```python
from build123d import *

# Parameters (mm, degrees)
SKETCH1_W            = 213.868
SKETCH1_H            = 49.53
BOSS_EXTRUDE1_DEPTH  = 63.5
SKETCH2_W            = 203.708
SKETCH2_H            = 39.37
CUT_EXTRUDE1_DEPTH   = 11.43
SKETCH3_W            = 191.008
SKETCH3_H            = 29.21
CUT_EXTRUDE2_DEPTH   = 45.72
SKETCH5_W            = 29.21
SKETCH5_H            = 45.72
BOSS_EXTRUDE2_DEPTH  = 31.75
SKETCH7_W            = 29.21
SKETCH7_H            = 45.802108617
BOSS_EXTRUDE3_DEPTH  = 31.75
BOSS_EXTRUDE4_DEPTH  = 40.64
BOSS_EXTRUDE5_DEPTH  = 40.64
SKETCH20_W           = 12.7
SKETCH20_H           = 29.21
BOSS_EXTRUDE6_DEPTH  = 18.542
BOSS_EXTRUDE7_DEPTH  = 30.48
SKETCH22_W           = 106.68
SKETCH22_H           = 63.5
BOSS_EXTRUDE8_DEPTH  = 26.67
CUT_EXTRUDE11_DEPTH  = 96.52
CUT_EXTRUDE5_DEPTH   = 49.53
SKETCH28_W           = 12.7
SKETCH28_H           = 29.21
CUT_EXTRUDE6_DEPTH   = 28.702
BOSS_EXTRUDE9_DEPTH  = 29.21
SKETCH30_W           = 12.7
SKETCH30_H           = 29.21
CUT_EXTRUDE7_DEPTH   = 28.702
BOSS_EXTRUDE11_DEPTH = 29.21
BOSS_EXTRUDE12_DEPTH = 29.21
CUT_EXTRUDE8_DEPTH   = 49.53
BOSS_EXTRUDE13_DEPTH = 29.21
CUT_EXTRUDE9_DEPTH   = 50.8
CUT_EXTRUDE12_DEPTH  = 49.53
SKETCH48_W           = 12.7
SKETCH48_H           = 5.334
BOSS_EXTRUDE14_DEPTH = 31.242
BOSS_EXTRUDE17_DEPTH = 31.242
SKETCH52_W           = 12.7
SKETCH52_H           = 5.334
BOSS_EXTRUDE18_DEPTH = 31.242
BOSS_EXTRUDE19_DEPTH = 31.242
SKETCH54_W           = 12.7
SKETCH54_H           = 5.334
BOSS_EXTRUDE20_DEPTH = 31.242
BOSS_EXTRUDE21_DEPTH = 31.242
SKETCH56_W           = 12.7
SKETCH56_H           = 5.334
BOSS_EXTRUDE22_DEPTH = 31.242
BOSS_EXTRUDE23_DEPTH = 31.242


with BuildPart() as part:
    # Sketch1 → Boss-Extrude1 (new body)
    with BuildSketch(Plane(origin=(0, 0, 0), x_dir=(1, 0, 0), z_dir=(0, 1, 0))):
        with Locations((47.373649513, -17.485904033)):
            Rectangle(SKETCH1_W, SKETCH1_H)
    extrude(amount=BOSS_EXTRUDE1_DEPTH)

    # Sketch2 → Cut-Extrude1 (cut)
    with BuildSketch(Plane(origin=(0, 63.5, 0), x_dir=(1, 0, 0), z_dir=(0, 1, 0))):
        with Locations((47.373649513, -17.485904033)):
            Rectangle(SKETCH2_W, SKETCH2_H)
    extrude(amount=-CUT_EXTRUDE1_DEPTH, mode=Mode.SUBTRACT)

    # Sketch3 → Cut-Extrude2 (cut)
    with BuildSketch(Plane(origin=(0, 52.07, 0), x_dir=(1, 0, 0), z_dir=(0, 1, 0))):
        with Locations((47.373649513, -17.485904033)):
            Rectangle(SKETCH3_W, SKETCH3_H)
    extrude(amount=-CUT_EXTRUDE2_DEPTH, mode=Mode.SUBTRACT)

    # Sketch5 → Boss-Extrude2 (add)
    with BuildSketch(Plane.ZY.offset(-142.877649513)):
        with Locations((17.485904033, 29.21)):
            Rectangle(SKETCH5_W, SKETCH5_H)
    extrude(amount=BOSS_EXTRUDE2_DEPTH)

    # Sketch7 → Boss-Extrude3 (add)
    with BuildSketch(Plane(origin=(-48.130350487, 0, 0), x_dir=(0, 0, -1), z_dir=(1, 0, 0))):
        with Locations((-17.485904033, 29.168945691)):
            Rectangle(SKETCH7_W, SKETCH7_H)
    extrude(amount=BOSS_EXTRUDE3_DEPTH)

    # Sketch13 → Boss-Extrude4 (add)
    with BuildSketch(Plane.XY.offset(-2.199095967)):
        Polygon((-54.480350487, 62.738), (-48.130350487, 52.07), (-54.480350487, 52.07), align=None)
    extrude(amount=BOSS_EXTRUDE4_DEPTH)

    # Sketch19 → Boss-Extrude5 (add)
    with BuildSketch(Plane(origin=(0, 0, 37.170904033), x_dir=(-1, 0, 0), z_dir=(0, 0, -1))):
        Polygon((-149.227649513, 62.738), (-142.877649513, 52.07), (-149.227649513, 52.07), align=None)
    extrude(amount=BOSS_EXTRUDE5_DEPTH)

    # Sketch20 → Boss-Extrude6 (add)
    with BuildSketch(Plane(origin=(0, 6.35, 0), x_dir=(1, 0, 0), z_dir=(0, 1, 0))):
        with Locations((47.373649513, -17.485904033)):
            Rectangle(SKETCH20_W, SKETCH20_H)
    extrude(amount=BOSS_EXTRUDE6_DEPTH)

    # Sketch21 → Boss-Extrude7 (add)
    with BuildSketch(Plane.XY.offset(2.880904033)):
        Polygon((66.423649513, 37.592), (28.323649513, 37.592), (33.403649513, 24.892), (41.023649513, 24.892), (53.723649513, 24.892), (61.343649513, 24.892), align=None)
    extrude(amount=BOSS_EXTRUDE7_DEPTH)

    # Sketch22 → Boss-Extrude8 (add)
    with BuildSketch(Plane(origin=(0, 0, -7.279095967), x_dir=(-1, 0, 0), z_dir=(0, 0, -1))):
        with Locations((-46.357649513, 31.75)):
            Rectangle(SKETCH22_W, SKETCH22_H)
    extrude(amount=BOSS_EXTRUDE8_DEPTH)

    # Sketch39 → Cut-Extrude11 (cut)
    with BuildSketch(Plane(origin=(99.697649513, 0, 0), x_dir=(0, 0, -1), z_dir=(1, 0, 0))):
        with BuildLine():
            Line((12.359095967, 50.8), (12.359095967, 6.35))
            Line((12.359095967, 6.35), (27.599095967, 6.35))
            Line((27.599095967, 6.35), (27.599095967, 50.8))
            add(Edge.make_bspline(
                [(12.359095967, 50.8), (19.979095967, 66.04), (27.599095967, 50.8)],
                knots=[0, 0, 0, 1, 1, 1], degree=2))
        make_face()
    extrude(amount=-CUT_EXTRUDE11_DEPTH, mode=Mode.SUBTRACT)

    # Sketch26 → Cut-Extrude5 (cut)
    with BuildSketch(Plane(origin=(0, 0, -7.279095967), x_dir=(-1, 0, 0), z_dir=(0, 0, -1))):
        Polygon((-154.307649513, 38.1), (-106.047649513, 0), (-154.307649513, 0), align=None)
    extrude(amount=-CUT_EXTRUDE5_DEPTH, mode=Mode.SUBTRACT)

    # Sketch28 → Cut-Extrude6 (cut)
    with BuildSketch(Plane(origin=(0, 52.07, 0), x_dir=(1, 0, 0), z_dir=(0, 1, 0))):
        with Locations((117.477649513, -17.485904033)):
            Rectangle(SKETCH28_W, SKETCH28_H)
    extrude(amount=-CUT_EXTRUDE6_DEPTH, mode=Mode.SUBTRACT)

    # Sketch29 → Boss-Extrude9 (add)
    with BuildSketch(Plane(origin=(0, 0, 32.090904033), x_dir=(-1, 0, 0), z_dir=(0, 0, -1))):
        Polygon((-123.827649513, 52.07), (-111.127649513, 23.368), (-123.827649513, 23.368), align=None)
    extrude(amount=BOSS_EXTRUDE9_DEPTH)

    # Sketch30 → Cut-Extrude7 (cut)
    with BuildSketch(Plane(origin=(0, 52.07, 0), x_dir=(1, 0, 0), z_dir=(0, 1, 0))):
        with Locations((-22.730350487, -17.485904033)):
            Rectangle(SKETCH30_W, SKETCH30_H)
    extrude(amount=-CUT_EXTRUDE7_DEPTH, mode=Mode.SUBTRACT)

    # Sketch31 → Boss-Extrude11 (add)
    with BuildSketch(Plane(origin=(0, 0, 32.090904033), x_dir=(-1, 0, 0), z_dir=(0, 0, -1))):
        Polygon((16.380350487, 23.368), (29.080350487, 52.07), (29.080350487, 23.368), align=None)
    extrude(amount=BOSS_EXTRUDE11_DEPTH)

    # Sketch33 → Boss-Extrude12 (add)
    with BuildSketch(Plane(origin=(0, 0, 32.090904033), x_dir=(-1, 0, 0), z_dir=(0, 0, -1))):
        Polygon((-111.127649513, 23.368), (-98.427649513, 6.35), (-111.127649513, 6.35), align=None)
    extrude(amount=BOSS_EXTRUDE12_DEPTH)

    # Sketch34 → Cut-Extrude8 (cut)
    with BuildSketch(Plane(origin=(0, 0, -7.279095967), x_dir=(-1, 0, 0), z_dir=(0, 0, -1))):
        Polygon((-154.307649513, 38.1), (-135.257649513, 38.1), (-106.047649513, 0), align=None)
    extrude(amount=-CUT_EXTRUDE8_DEPTH, mode=Mode.SUBTRACT)

    # Sketch35 → Boss-Extrude13 (add)
    with BuildSketch(Plane(origin=(0, 0, 32.090904033), x_dir=(-1, 0, 0), z_dir=(0, 0, -1))):
        Polygon((16.380350487, 23.368), (3.680350487, 6.35), (16.380350487, 6.35), align=None)
    extrude(amount=BOSS_EXTRUDE13_DEPTH)

    # Sketch37 → Cut-Extrude9 (cut)
    with BuildSketch(Plane(origin=(0, 0, -7.279095967), x_dir=(-1, 0, 0), z_dir=(0, 0, -1))):
        Polygon((13.332350487, 0), (59.560350487, 38.1), (59.560350487, 0), align=None)
    extrude(amount=-CUT_EXTRUDE9_DEPTH, mode=Mode.SUBTRACT)

    # Sketch40 → Cut-Extrude12 (cut)
    with BuildSketch(Plane(origin=(0, 0, -7.279095967), x_dir=(-1, 0, 0), z_dir=(0, 0, -1))):
        Polygon((40.510350487, 38.1), (59.560350487, 38.1), (13.332350487, 0), align=None)
    extrude(amount=-CUT_EXTRUDE12_DEPTH, mode=Mode.SUBTRACT)

    # Sketch48 → Boss-Extrude14 (add)
    with BuildSketch(Plane(origin=(0, 6.35, 0), x_dir=(1, 0, 0), z_dir=(0, 1, 0))):
        with Locations((34.673649513, -5.547904033)):
            Rectangle(SKETCH48_W, SKETCH48_H)
    extrude(amount=BOSS_EXTRUDE14_DEPTH)

    # Sketch51 → Boss-Extrude17 (add)
    with BuildSketch(Plane(origin=(0, 6.35, 0), x_dir=(1, 0, 0), z_dir=(0, 1, 0))):
        Polygon((14.861649513, -2.880904033), (28.323649513, -8.214904033), (28.323649513, -2.880904033), align=None)
    extrude(amount=BOSS_EXTRUDE17_DEPTH)

    # Sketch52 → Boss-Extrude18 (add)
    with BuildSketch(Plane(origin=(0, 6.35, 0), x_dir=(1, 0, 0), z_dir=(0, 1, 0))):
        with Locations((34.673649513, -29.423904033)):
            Rectangle(SKETCH52_W, SKETCH52_H)
    extrude(amount=BOSS_EXTRUDE18_DEPTH)

    # Sketch53 → Boss-Extrude19 (add)
    with BuildSketch(Plane(origin=(0, 6.35, 0), x_dir=(1, 0, 0), z_dir=(0, 1, 0))):
        Polygon((14.861649513, -32.090904033), (28.323649513, -26.756904033), (28.323649513, -32.090904033), align=None)
    extrude(amount=BOSS_EXTRUDE19_DEPTH)

    # Sketch54 → Boss-Extrude20 (add)
    with BuildSketch(Plane(origin=(0, 6.35, 0), x_dir=(1, 0, 0), z_dir=(0, 1, 0))):
        with Locations((60.073649513, -5.547904033)):
            Rectangle(SKETCH54_W, SKETCH54_H)
    extrude(amount=BOSS_EXTRUDE20_DEPTH)

    # Sketch55 → Boss-Extrude21 (add)
    with BuildSketch(Plane(origin=(0, 6.35, 0), x_dir=(1, 0, 0), z_dir=(0, 1, 0))):
        Polygon((66.423649513, -8.214904033), (79.885649513, -2.880904033), (66.423649513, -2.880904033), align=None)
    extrude(amount=BOSS_EXTRUDE21_DEPTH)

    # Sketch56 → Boss-Extrude22 (add)
    with BuildSketch(Plane(origin=(0, 6.35, 0), x_dir=(1, 0, 0), z_dir=(0, 1, 0))):
        with Locations((60.073649513, -29.423904033)):
            Rectangle(SKETCH56_W, SKETCH56_H)
    extrude(amount=BOSS_EXTRUDE22_DEPTH)

    # Sketch57 → Boss-Extrude23 (add)
    with BuildSketch(Plane(origin=(0, 6.35, 0), x_dir=(1, 0, 0), z_dir=(0, 1, 0))):
        Polygon((66.423649513, -26.756904033), (79.885649513, -32.090904033), (66.423649513, -32.090904033), align=None)
    extrude(amount=BOSS_EXTRUDE23_DEPTH)


solid = part.part
```
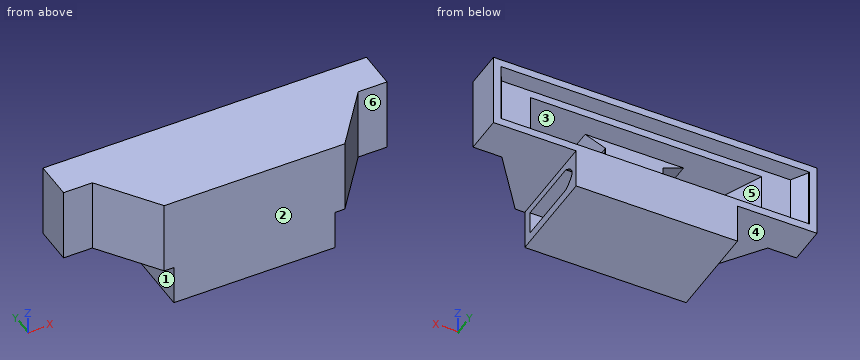
Design review of the part built by this model. Coordinates are the model's own, in mm. Face numbers are marked on the shaded views. A direction names the side the tool comes from. Give positions to 0.01 mm unless a question says otherwise; leave off trailing zeros. Loops run counter-clockwise (first coordinate to the right, second up) from the corner with the lowest first, then second, coordinate; pieces in that order, holes last. Notation, with made-up numbers: M 48.5,5 L 104.5,5 A25 ccw 104.5,30 Z; hole C 37,-21.5 d9. An arc over 180 degrees is marked long. Return JSON: item names as keys, results as strings. Group by question number.
Item 1: Tool access review of the marked faces 4, 5 and 6: name each direction out of +Z, -Z, +X, -X, +Y, -Y from which nothing blocks a thin tool from reaching the whole face with its end or side.
Item 2: Mouldability with a two-part tool opening along X and no side actions: class the marked faces 1, 2 and 3 as released by +X, released by -X, zero draft, split by the parting line, or undercut.
Item 3: We need section C-C (z = 19). Give the boundary of the cut face in (x, y).
Item 4: For probe 1 along Z at (x, y) = (11, 50); probe 2 along Z at (x, y) = (34.5, 60.5); probe 3 along Z at (x, y) = (61.5, 21.5), list the stretches that pass through material, from the lowest coordinate up.
Item 5: We need section B-B (x = 113.5). Give the boundary of the cut face in (y, z), and give its area (3 significant figures).
Item 6: Insertion check: pin 1 Ø21.5 at (y, z) = (38, -27) entering from -X; pin 2 Ø12 at (x, y) = (109, 53.5) entering from -Z; pin 3 Ø12 at (y, z) = (26, -6.5) entering from +X. Each pin has a flat end and moves straight along its axis. Give the tip position at first contact, or say it passes through.
Item 7: We need section D-D (x = 36). Give the number of separate pieces and of enclosed holes in the cut face, and give its area (3 significant figures).
Item 8: We need section A-A (y = 45). Give the boundary of the cut face in (x, z), and give its area (3 significant figures).
Output:
{
 "1": {"face 4": "-Z, -X, +Y, -Y", "face 5": "+Y", "face 6": "+Z, -Z, +X, -Y"},
 "2": {"face 1": "released by -X", "face 2": "zero draft", "face 3": "undercut"},
 "3": {"outline": "M -59.56,38.1 L -40.51,38.1 L -13.33,0 L 106.05,0 L 135.26,38.1 L 154.31,38.1 L 154.31,63.5 L 149.23,63.5 L 149.23,62.74 L 142.88,52.07 L 123.83,52.07 L 111.13,23.37 L 98.43,6.35 L 53.72,6.35 L 53.72,24.89 L 61.34,24.89 L 66.42,37.59 L 28.32,37.59 L 33.4,24.89 L 41.02,24.89 L 41.02,6.35 L -3.68,6.35 L -16.38,23.37 L -29.08,52.07 L -48.13,52.07 L -54.48,62.74 L -54.48,63.5 L -59.56,63.5 Z"},
 "4": {"probe 1": "z = -33.95 to -27.6, -12.36 to 2.88, 32.09 to 42.25", "probe 2": "z = -33.95 to -2.2, 37.17 to 42.25", "probe 3": "z = -33.95 to -27.6, -12.36 to 8.21, 26.76 to 42.25"},
 "5": {"outline": "M 9.72,-7.28 L 63.5,-7.28 L 63.5,-2.2 L 52.07,-2.2 L 52.07,2.88 L 28.73,2.88 L 28.73,32.09 L 52.07,32.09 L 52.07,37.17 L 63.5,37.17 L 63.5,42.25 L 9.72,42.25 Z", "area": "1,530 mm^2"},
 "6": {"pin 1": "stops at x = -6.98", "pin 2": "stops at z = -7.28", "pin 3": "stops at x = 130.58"},
 "7": {"separate pieces": "1", "enclosed holes": "2", "area": "2,870 mm^2"},
 "8": {"outline": "M -59.56,-7.28 L -6.98,-7.28 L -6.98,-33.95 L 99.7,-33.95 L 99.7,-27.6 L 3.18,-27.6 L 3.18,-12.36 L 99.7,-12.36 L 99.7,-7.28 L 154.31,-7.28 L 154.31,42.25 L -59.56,42.25 Z; hole M -25.95,2.88 L 120.7,2.88 L 120.7,32.09 L -25.95,32.09 Z", "area": "7,680 mm^2"}
}
